from build123d import *

# Parameters (mm, degrees)
F0_W     = 77
F0_H     = 20
F1_DEPTH = 10
F2_W     = 67
F2_H     = 16
F3_DEPTH = 8
F7_R     = 1
F8_DEPTH = 25


with BuildPart() as f1:
    # F0 (on Top) → F1 (new body)
    with BuildSketch(Plane.XY):
        Rectangle(F0_W, F0_H)
    extrude(amount=F1_DEPTH)

    # F2 (on face) → F3 (cut)
    with BuildSketch(Plane.XY.offset(10)):
        Rectangle(F2_W, F2_H)
    extrude(amount=-F3_DEPTH, mode=Mode.SUBTRACT)


with BuildPart() as f5_1:
    # F5: instance of F1
    add(f1.part.mirror(Plane.XY.offset(25)))

    # F7 (on face) → F8 (cut)
    with BuildSketch(Plane(origin=(0, 0, 40), x_dir=(1, 0, 0), z_dir=(0, 0, -1))):
        with Locations((36, 0)):
            Circle(F7_R)
        with Locations((-36, 0)):
            Circle(F7_R)
    extrude(amount=-F8_DEPTH, mode=Mode.SUBTRACT)


solid = f5_1.part
Geometry check sheet. Reference: the model listing, model coordinates, mm. A direction names the side the tool comes from. Round coordinates to 2 decimals unless told otherwise and drop trailing zeros. Loops run counter-clockwise (first coordinate to the right, second up) from the corner with the lowest first, then second, coordinate; pieces in that order, holes last. Notation, with made-up numbers: (15, -33) - (50, -33) arc R26 ccw to (50, -9) - close; hole circle Ø10 at (-31, 87). An arc over 180 degrees is marked (long way). Answer as CSV lines item,"result".
(1) Release check for a two-part mould opening along Y. For faces 3 (the face through (-1, -10, 45)), 4 (the face through (-1, -9, 40)), 5 (the face through (33.5, 0, 44)) record: released by +Y, released by -Y, zero draft, split by the parting line, or undercut.
Output values:
face 3,"released by -Y"
face 4,"zero draft"
face 5,"undercut"
(2) Cross-section at C-C, the plane z = 41.5. Enter the section's corners in (x, y), and give its area (3 significant figures).
Output values:
outline,"(-38.5, -10) - (38.5, -10) - (38.5, 10) - (-38.5, 10) - close; hole circle Ø2 at (-36, 0); hole (-33.5, -8) - (33.5, -8) - (33.5, 8) - (-33.5, 8) - close; hole circle Ø2 at (36, 0)"
area,"462 mm²"
(3) Depth check by flat-ended pin: pin 1 Ø5 at (x, y) = (-11, -1) entering from -Z; pin 2 Ø1.6 at (x, y) = (36, 0) entering from +Z. Enter the tip coordinate at first touch or a pass-through.
Output values:
pin 1,"stops at z = 48"
pin 2,"passes through"
(4) Cross-section at A-A, the plane x = 36. Enter the section's corners in (y, z).
Output values:
outline,"(-10, 40) - (-1, 40) - (-1, 50) - (-10, 50) - close; (1, 40) - (10, 40) - (10, 50) - (1, 50) - close"
(5) Material ranges on line 1 along X through (y, z) = (0, 42.5); line 2 along Y through (x, z) = (30, 41.25); line 3 along X through (y, z) = (-6.5, 46.75), recorded low to high.
Output values:
line 1,"x = -38.5 to -37, -35 to -33.5, 33.5 to 35, 37 to 38.5"
line 2,"y = -10 to -8, 8 to 10"
line 3,"x = -38.5 to -33.5, 33.5 to 38.5"
(6) Set-up check for faces 1 (the face through (0, -8, 44)), 2 (the face through (-1, 10, 45)): record each of +Z, -Z, +X, -X, +Y, -Y from which the full face is reachable in a straight line by a thin tool's end or side.
Output values:
face 1,"-Z"
face 2,"+Z, -Z, +X, -X, +Y"
(7) Cross-section at D-D, the plane y = -5. Enter the section's corners in (x, z), and give its area (3 significant figures).
Output values:
outline,"(-38.5, 40) - (-33.5, 40) - (-33.5, 48) - (33.5, 48) - (33.5, 40) - (38.5, 40) - (38.5, 50) - (-38.5, 50) - close"
area,"234 mm²"
(8) Cross-section at B-B, the plane y = 0. Enter the section's corners in (x, z), and give its area (3 significant figures).
Output values:
outline,"(-38.5, 40) - (-37, 40) - (-37, 50) - (-38.5, 50) - close; (-35, 40) - (-33.5, 40) - (-33.5, 48) - (33.5, 48) - (33.5, 40) - (35, 40) - (35, 50) - (-35, 50) - close; (37, 40) - (38.5, 40) - (38.5, 50) - (37, 50) - close"
area,"194 mm²"
